from build123d import *

# Parameters (mm, degrees)
CHAMFER1_SIZE = 0.5


with BuildPart() as part:
    # Sketch2 → Revolve1 (revolve)
    with BuildSketch(Plane.XY, mode=Mode.PRIVATE) as revolve1_sk:
        Polygon((12.4079, -3.75), (10.4079, -3.75), (10.4079, 0), (0, 0), (0, 2), (13.4079, 2), (13.4079, 1.05), (12.4079, 1.05), align=None)
    revolve(revolve1_sk.sketch.rotate(Axis((0, 0, 0), (0, 1, 0)), 90), axis=Axis((0, 0, 0), (0, 1, 0)))  # turned: the seam where the file's is

    # Chamfer1
    chamfer1_edges = [part.edges().sort_by_distance(p)[0] for p in [
        (0, -3.75, 12.4079),
        (0, 2, 13.4079),
    ]]
    chamfer(chamfer1_edges, length=CHAMFER1_SIZE)


solid = part.part
Could you check a few things on this model? Use its own coordinates, in mm. A direction names the side the tool comes from. Coordinates: 2 decimals unless noted, no trailing zeros. Order: outer loops, then holes, each group sorted by start corner. A loop starts at its lowest first (then second) coordinate and runs counter-clockwise, first axis right, second up. Notation, with made-up numbers: (-24, -0.75) - (2, -0.75) arc R15 cw to (2, 10.25) - close; hole circle Ø4 at (62.25, 65). An arc over 180 degrees is marked (long way). Answer in a Markdown table with one row per item. Add a question column.
(1) If we mould it in two halves opening along Z, with no side actions, what happens to faces 3 (the face through (-9.062, 1.272, 9.882)), 4 (the face through (0, 0, 0)), 5 (the face through (0, 2, 0))? For each: released by +Z, released by -Z, zero draft, split by the parting line, or undercut.
(2) I need wall thicknesses on L1, parallel to X at y = -0.8, z = 0; L2, parallel to Y at x = -1.5, z = -1; L3, parallel to X at y = -1.8, z = -8.5. Which ranges of each line are inside material? Lowest first, please.
(3) If we section it at C-C, the plane y = -0.5: Please give me the cut outline in (x, z).
(4) If we section it at B-B, the plane z = 0: Please give me the cut outline in (x, y).
(5) Will these pins go through, and if not, where does the flat tip stop? pin 1 (1 mm diameter, centred on x = 7, y = -1.5, fed in from +Z); pin 2 (3 mm diameter, centred on y = -1, z = 3.5, fed in from +X).
(6) If we section it at A-A, the plane x = 0: Please give me the cut outline in (y, z), then the cut area to 3 significant figures.
(7) On a 3-axis mill with a long thin cutter (end or side, diameter ignored), from which of +Z, -Z, +X, -X, +Y, -Y can I reach the whole of each face in a straight line? I mean faces 1 (the face through (12, 1.05, -4)), 2 (the face through (11, -3.75, 0)). Say none if no direction works.
Results are:
| question | item | result |
|---|---|---|
| 1 | face 3 | split by the parting line |
| 1 | face 4 | undercut |
| 1 | face 5 | zero draft |
| 2 | L1 | x = -12.41 to -10.41, 10.41 to 12.41 |
| 2 | L2 | y = 0 to 2 |
| 2 | L3 | x = -9.04 to -6.01, 6.01 to 9.04 |
| 3 | outline | circle Ø24.82 at (0, 0); hole circle Ø20.82 at (0, 0) |
| 4 | outline | (-13.41, 1.05) - (-12.41, 1.05) - (-12.41, -3.25) - (-11.91, -3.75) - (-10.41, -3.75) - (-10.41, 0) - (10.41, 0) - (10.41, -3.75) - (11.91, -3.75) - (12.41, -3.25) - (12.41, 1.05) - (13.41, 1.05) - (13.41, 1.5) - (12.91, 2) - (-12.91, 2) - (-13.41, 1.5) - close |
| 5 | pin 1 | stops at z = 10.57 |
| 5 | pin 2 | stops at x = 12.25 |
| 6 | outline | (-3.75, -11.91) - (-3.25, -12.41) - (1.05, -12.41) - (1.05, -13.41) - (1.5, -13.41) - (2, -12.91) - (2, 12.91) - (1.5, 13.41) - (1.05, 13.41) - (1.05, 12.41) - (-3.25, 12.41) - (-3.75, 11.91) - (-3.75, 10.41) - (0, 10.41) - (0, -10.41) - (-3.75, -10.41) - close |
| 6 | area | 66.0 mm2 |
| 7 | face 1 | -Y |
| 7 | face 2 | +Z, -Z, +X, -X, -Y |
